Geometry: final body of the model. Coordinates: model frame, mm. Face numbers are marked on the shaded views. A direction names the side the tool comes from. Round coordinates to 2 decimals unless told otherwise and drop trailing zeros. Order: outer loops, then holes, each group sorted by start corner. A loop starts at its lowest first (then second) coordinate and runs counter-clockwise, first axis right, second up. Notation, with made-up numbers: (-6.75, -35) - (6.25, -35) arc R22 cw to (6.25, 3) - close; hole circle Ø4 at (39.25, 15). An arc over 180 degrees is marked (long way). Put each result on its own line as item: value. Start each with the question number.
(1) Section D-D (x = 28). Output: boundary loops of the cut face in (y, z).
(2) Material intervals for L1, parallel to Z at x = 118, y = -128.45; L2, parallel to Z at x = 69, y = -127; L3, parallel to Z at x = 118, y = -129, sorted ascending. Write a range as [from, to].
(3) Section A-A (x = 118). Output: boundary loops of the cut face in (y, z).
(4) Section C-C (z = 58). Output: boundary loops of the cut face in (x, y).
(5) Access query for the marked faces 1 and 2. Directions: +Z, -Z, +X, -X, +Y, -Y. A direction counts if a zero-diameter tool reaches every point of the face in a straight line with its end or side. Return the directions, or none.
(6) Section B-B (y = -68). Output: boundary loops of the cut face in (x, z), and give its area (3 significant figures).
(7) Pin query (flat end, axial travel): P1, Ø6.5, axis at x = 118, z = 58, coming from the +Y side; P2, Ø2.5, axis at x = 14.5, z = 58, coming from the +Y side; P3, Ø4, axis at x = 105.5, z = 58, coming from the +Y side; P4, Ø3, axis at x = 55.5, y = -27, coming from the +Z side. Return the tip coordinate at first contact, or that it passes through.
from build123d import *

# Parameters (mm, degrees)
F1_DEPTH  = 133
F2_R      = 2.5
F3_DEPTH  = 25
F4_R      = 4
F5_DEPTH  = 5
F6_DEPTH  = 25
F7_R      = 3
F9_DEPTH  = 25
F11_DEPTH = 2
F13_DEPTH = 2


with BuildPart() as f1:
    # F0 (on Right) → F1 (new body)
    with BuildSketch(Plane.YZ):
        Polygon((-128.955605, 0), (-128.955605, 110), (-130.955605, 110), (-130.955605, 0), (-130.955605, -2), (46.044395, -2), (46.044395, 0), align=None)
    extrude(amount=F1_DEPTH)

    # F2 (on face) → F3 (cut)
    with BuildSketch(Plane.XZ.offset(130.955605)):
        with Locations((69, 13)):
            Circle(F2_R)
        with Locations((15, 58)):
            Circle(F2_R)
        with Locations((118, 58)):
            Circle(F2_R)
    extrude(amount=-F3_DEPTH, mode=Mode.SUBTRACT)

    # F4 (on face) → F5 (join)
    with BuildSketch(Plane.XZ.offset(130.955605)):
        with Locations((15, 58)):
            Circle(F4_R)
        with Locations((69, 13)):
            Circle(F4_R)
        with Locations((118, 58)):
            Circle(F4_R)
    extrude(amount=-F5_DEPTH)

    # F2 (on face) → F6 (cut)
    with BuildSketch(Plane.XZ.offset(130.955605)):
        with Locations((69, 13)):
            Circle(F2_R)
        with Locations((15, 58)):
            Circle(F2_R)
        with Locations((118, 58)):
            Circle(F2_R)
    extrude(amount=-F6_DEPTH, mode=Mode.SUBTRACT)

    # F7
    f7_edges = [f1.edges().sort_by_distance(p)[0] for p in [
        (0, -129.955605, 110),
        (133, -129.955605, 110),
        (133, 46.044395, -1),
        (0, 46.044395, -1),
    ]]
    fillet(f7_edges, radius=F7_R)

    # F8 (on face) → F9 (cut)
    with BuildSketch(Plane.XY):
        with BuildLine():
            Line((64, 7.044395), (64, -92.955605))
            ThreePointArc((64, -92.955605), (66.5, -95.455605), (69, -92.955605))
            Line((69, -92.955605), (69, 7.044395))
            ThreePointArc((69, 7.044395), (66.5, 9.544395), (64, 7.044395))
        make_face()
    extrude(amount=-F9_DEPTH, mode=Mode.SUBTRACT)

    # F10 (on face) → F11 (join)
    with BuildSketch(Plane.YZ.offset(133)):
        with BuildLine():
            Line((-130.955605, 109.6), (-130.955605, -2))
            Line((-130.955605, -2), (-30.955605, -2))
            ThreePointArc((-30.955605, -2), (-89.169777, 46.439631), (-130.955605, 109.6))
        make_face()
    extrude(amount=-F11_DEPTH)

    # F12 (on face) → F13 (join)
    with BuildSketch(Plane(origin=(0, 0, 0), x_dir=(0, -1, 0), z_dir=(-1, 0, 0))):
        with BuildLine():
            Line((30.955605, -2), (130.955605, -2))
            Line((130.955605, -2), (130.955605, 109.6))
            ThreePointArc((130.955605, 109.6), (89.169777, 46.439631), (30.955605, -2))
        make_face()
    extrude(amount=-F13_DEPTH)


solid = f1.part
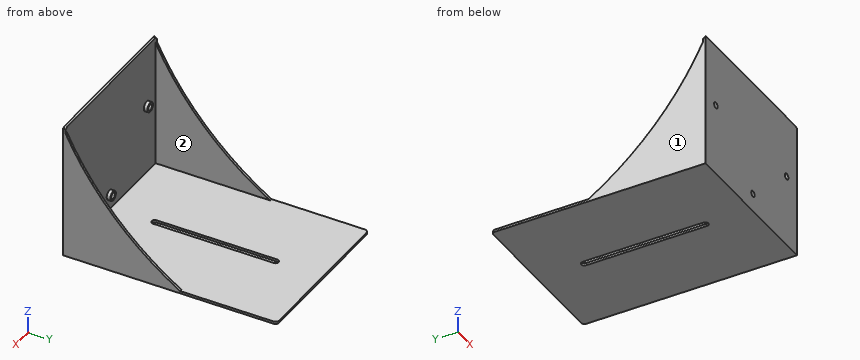
Checks:
1. outline: (-130.96, -2) - (46.04, -2) - (46.04, 0) - (-128.96, 0) - (-128.96, 110) - (-130.96, 110) - close
2. L1: z = [-2, 0], [54, 55.5], [60.5, 62]
2. L2: z = [-2, 0], [9, 10.5], [15.5, 17]
2. L3: z = [-2, 55.5], [60.5, 110]
3. outline: (-130.96, -2) - (46.04, -2) - (46.04, 0) - (-128.96, 0) - (-128.96, 54) - (-125.96, 54) - (-125.96, 55.5) - (-130.96, 55.5) - close; (-130.96, 60.5) - (-125.96, 60.5) - (-125.96, 62) - (-128.96, 62) - (-128.96, 110) - (-130.96, 110) - close
4. outline: (0, -130.96) - (12.5, -130.96) - (12.5, -125.96) - (11, -125.96) - (11, -128.96) - (2, -128.96) - (2, -98.94) - (0, -98.94) - close; (17.5, -130.96) - (115.5, -130.96) - (115.5, -125.96) - (114, -125.96) - (114, -128.96) - (19, -128.96) - (19, -125.96) - (17.5, -125.96) - close; (120.5, -130.96) - (133, -130.96) - (133, -98.94) - (131, -98.94) - (131, -128.96) - (122, -128.96) - (122, -125.96) - (120.5, -125.96) - close
5. face 1: +Z, -Z, -X, +Y, -Y
5. face 2: +Z, +Y
6. outline: (0, -2) - (64, -2) - (64, 0) - (2, 0) - (2, 25.38) - (0, 25.38) - close; (69, -2) - (133, -2) - (133, 25.38) - (131, 25.38) - (131, 0) - (69, 0) - close
6. area: 358 mm²
7. P1: stops at y = -125.96
7. P2: passes through
7. P3: stops at y = -128.96
7. P4: stops at z = 0
